Design review of the part built by this model. Coordinates are the model's own, in mm. A direction names the side the tool comes from. Coordinates: 2 decimals unless noted, no trailing zeros. Loops run counter-clockwise (first coordinate to the right, second up) from the corner with the lowest first, then second, coordinate; pieces in that order, holes last. Notation, with made-up numbers: M -35.75,-15.5 L -28.75,-15.5 A17 ccw -28.75,-11.5 Z; hole C 9,2.25 d4. An arc over 180 degrees is marked long. Answer as a JSON object with one key per item and string values. Group by question number.
1. Draft analysis for pull direction Y (two halves, no side actions). For faces 6 (the conical face through (-9.51, 40.769, -2.812)), 7 (the cylindrical face through (-1.97, -27.01, -24.85)), 8 (the flat face through (-20.3, 30, -2)), state which applies: +Y half, -Y half, draft (parallel to the pull), parting line (faces both ways), or undercut.
2. To check wall thickness, follow probe 1 along X at (y, z) = (-3.3, -10.15); probe 2 along X at (y, z) = (-3.5, -46); probe 3 along Z at (x, y) = (-19.5, 35). State the ranges of each line that lie inside material, in increasing order.
3. Consider section C-C (z = -17.5). State the section outline as (x, y) points, then the cut area to 3 significant figures.
4. Machinability: for faces 1 (the flat face through (-42, -24, -2)), 2 (the flat face through (-4, -31, -18)), 3 (the flat face through (-14, 25, -4)), 4 (the flat face through (-2, 30, -22)), 5 (the flat face through (-2, -24, -43)), which of the approach directions +Z, -Z, +X, -X, +Y, -Y give a long, thin tool a straight path to every point of the face, cutting with its end or side? Answer none if there is none.
5. Consider section B-B (x = -32). State the section outline as (y, z) points, then the cut area to 3 significant figures.
6. Insertion check: pin 1 (2 mm diameter, centred on x = -14.5, z = -8, fed in from -Y); pin 2 (1.2 mm diameter, centred on x = -10.15, z = -46, fed in from -Y); pin 3 (2.5 mm diameter, centred on x = -9.5, y = 42, fed in from +Z); pin 4 (12 mm diameter, centred on x = -16.5, y = -45, fed in from -Z). Each pin has a flat end and moves straight along its axis. Give the tip position at first contact, or say it passes through.
7. Consider section A-A (z = -38.5). State the section outline as (x, y) points, then the cut area to 3 significant figures.
from build123d import *

# Parameters (mm, degrees)
SKETCH1_W                    = 33.7
SKETCH1_H                    = 20.3
SKETCH1_W_2                  = 20.3
SKETCH1_H_2                  = 33.7
BOSS_EXTRUDE1_DEPTH          = 24
SHELL1_T                     = -4
SKETCH2_R                    = 1
CUT_EXTRUDE1_DEPTH           = 24
SKETCH3_R                    = 4.2
CUT_EXTRUDE2_DEPTH           = 3
CUT_EXTRUDE2_DRAFT           = -45
CUT_EXTRUDE2_PROFILE_2_DEPTH = 3
CUT_EXTRUDE2_PROFILE_2_DRAFT = -45
SKETCH4_W                    = 20.3
SKETCH4_H                    = 22
BOSS_EXTRUDE2_DEPTH          = 50
SHELL2_T                     = -4
CUT_EXTRUDE3_REACH           = 93.28
SKETCH5_R                    = 1
SKETCH6_R                    = 4.2
CUT_EXTRUDE4_DEPTH           = 3
CUT_EXTRUDE4_DRAFT           = -45
CUT_EXTRUDE5_REACH           = 93.28
SKETCH7_R                    = 1
SKETCH8_R                    = 4.2
CUT_EXTRUDE6_DEPTH           = 3
CUT_EXTRUDE6_DRAFT           = -45
FILLET1_R                    = 10
BOSS_EXTRUDE3_DEPTH          = 50
MIRROR4_COPY_1_SKETCH_R      = 4.2
MIRROR4_COPY_1_DEPTH         = 3
MIRROR4_COPY_1_DRAFT         = -45
MIRROR4_COPY_2_SKETCH_R      = 4.2
MIRROR4_COPY_2_DEPTH         = 3
MIRROR4_COPY_2_DRAFT         = -45
FILLET2_R                    = 10


with BuildPart() as part:
    # Sketch1 → Boss-Extrude1 (new body)
    with BuildSketch(Plane(origin=(0, 0, 0), x_dir=(1, 0, 0), z_dir=(0, 1, 0))):
        with Locations((-37.15, 10.15)):
            Rectangle(SKETCH1_W, SKETCH1_H)
        with Locations((-10.15, 10.15)):
            Rectangle(SKETCH1_W_2, SKETCH1_H)
        with Locations((-10.15, 37.15)):
            Rectangle(SKETCH1_W_2, SKETCH1_H_2)
    extrude(amount=-BOSS_EXTRUDE1_DEPTH)

    # Shell1
    shell1_openings = [part.faces().sort_by_distance(p)[0] for p in [
        (-53.236324676, -24, -10.15),
        (-54, -12, -10.15),
        (-37.15, -12, -20.3),
        (-20.3, -12, -37.15),
        (-10.15, -12, -54),
    ]]
    offset(amount=SHELL1_T, openings=shell1_openings, kind=Kind.INTERSECTION)

    # Sketch2 → Cut-Extrude1 (cut)
    with BuildSketch(Plane(origin=(0, 0, 0), x_dir=(1, 0, 0), z_dir=(0, 1, 0))):
        with Locations(Location((-10.15, 46, 0), (0, 0, 270))):
            Circle(SKETCH2_R)
        with Locations(Location((-46, 10.15, 0), (0, 0, 270))):
            Circle(SKETCH2_R)
    extrude(amount=-CUT_EXTRUDE1_DEPTH, mode=Mode.SUBTRACT)


with BuildPart() as cut_extrude2_tool:
    # Sketch3 → Cut-Extrude2 (with draft: the straight prism first)
    with BuildSketch(Plane(origin=(0, 0, 0), x_dir=(1, 0, 0), z_dir=(0, 1, 0))):
        with Locations((-46, 10.15)):
            Circle(SKETCH3_R)
    extrude(amount=-CUT_EXTRUDE2_DEPTH)
    # Cut-Extrude2: the draft: its side faces are tilted about the plane it starts from
    cut_extrude2_sides = [cut_extrude2_tool.faces().sort_by_distance(p)[0] for p in [
        (-50.2, -1.5, -10.15),
    ]]
    draft(cut_extrude2_sides, Plane(origin=(0, 0, 0), x_dir=(1, 0, 0), z_dir=(0, 1, 0)), CUT_EXTRUDE2_DRAFT)


with BuildPart() as part_1:
    add(part.part)

    # Cut-Extrude2: cut by cut_extrude2_tool
    add(cut_extrude2_tool.part, mode=Mode.SUBTRACT)


with BuildPart() as cut_extrude2_profile_2_tool:
    # Sketch3 → Cut-Extrude2 profile 2 (with draft: the straight prism first)
    with BuildSketch(Plane(origin=(0, 0, 0), x_dir=(1, 0, 0), z_dir=(0, 1, 0))):
        with Locations((-10.15, 46)):
            Circle(SKETCH3_R)
    extrude(amount=-CUT_EXTRUDE2_PROFILE_2_DEPTH)
    # Cut-Extrude2 profile 2: the draft: its side faces are tilted about the plane it starts from
    cut_extrude2_profile_2_sides = [cut_extrude2_profile_2_tool.faces().sort_by_distance(p)[0] for p in [
        (-14.35, -1.5, -46),
    ]]
    draft(cut_extrude2_profile_2_sides, Plane(origin=(0, 0, 0), x_dir=(1, 0, 0), z_dir=(0, 1, 0)), CUT_EXTRUDE2_PROFILE_2_DRAFT)


with BuildPart() as part_2:
    add(part_1.part)

    # Cut-Extrude2 profile 2: cut by cut_extrude2_profile_2_tool
    add(cut_extrude2_profile_2_tool.part, mode=Mode.SUBTRACT)


with BuildPart() as body_2:
    # Sketch4 → Boss-Extrude2 (new body)
    with BuildSketch(Plane(origin=(0, 0, 0), x_dir=(1, 0, 0), z_dir=(0, 1, 0))):
        with Locations((-10.15, 11)):
            Rectangle(SKETCH4_W, SKETCH4_H)
    extrude(amount=BOSS_EXTRUDE2_DEPTH)

    # Shell2
    shell2_openings = [body_2.faces().sort_by_distance(p)[0] for p in [
        (-10.15, 50, -11),
        (-10.15, 0, -11),
        (-20.3, 25, -11),
        (-10.15, 25, -22),
    ]]
    offset(amount=SHELL2_T, openings=shell2_openings, kind=Kind.INTERSECTION)


with BuildPart() as part_3:
    add(part_2.part)

    # Combine1: union body 2
    add(body_2.part)

    # Sketch5 → Cut-Extrude3 (cut, up to next)
    with BuildSketch(Plane.XY, mode=Mode.PRIVATE) as cut_extrude3_sk1:
        with Locations((-10.15, 42)):
            Circle(SKETCH5_R)
    cut_extrude3_tool1 = extrude(cut_extrude3_sk1.sketch, amount=-CUT_EXTRUDE3_REACH, mode=Mode.PRIVATE) & part_3.part
    cut_extrude3 = cut_extrude3_tool1.solids().sort_by_distance((-10.15, 42, 0))[0]
    add(cut_extrude3, mode=Mode.SUBTRACT)


with BuildPart() as cut_extrude4_tool:
    # Sketch6 → Cut-Extrude4 (with draft: the straight prism first)
    with BuildSketch(Plane.XY):
        with Locations((-10.15, 42)):
            Circle(SKETCH6_R)
    extrude(amount=-CUT_EXTRUDE4_DEPTH)
    # Cut-Extrude4: the draft: its side faces are tilted about the plane it starts from
    cut_extrude4_sides = [cut_extrude4_tool.faces().sort_by_distance(p)[0] for p in [
        (-14.35, 42, -1.5),
    ]]
    draft(cut_extrude4_sides, Plane.XY, CUT_EXTRUDE4_DRAFT)


with BuildPart() as part_4:
    add(part_3.part)

    # Cut-Extrude4: cut by cut_extrude4_tool
    add(cut_extrude4_tool.part, mode=Mode.SUBTRACT)

    # Sketch7 → Cut-Extrude5 (cut, up to next)
    with BuildSketch(Plane(origin=(0, 0, 0), x_dir=(0, 0, -1), z_dir=(1, 0, 0)), mode=Mode.PRIVATE) as cut_extrude5_sk1:
        with Locations((11, 20)):
            Circle(SKETCH7_R)
    cut_extrude5_tool1 = extrude(cut_extrude5_sk1.sketch, amount=-CUT_EXTRUDE5_REACH, mode=Mode.PRIVATE) & part_4.part
    cut_extrude5 = cut_extrude5_tool1.solids().sort_by_distance((0, 20, -11))[0]
    add(cut_extrude5, mode=Mode.SUBTRACT)


with BuildPart() as cut_extrude6_tool:
    # Sketch8 → Cut-Extrude6 (with draft: the straight prism first)
    with BuildSketch(Plane(origin=(0, 0, 0), x_dir=(0, 0, -1), z_dir=(1, 0, 0))):
        with Locations((11, 20)):
            Circle(SKETCH8_R)
    extrude(amount=-CUT_EXTRUDE6_DEPTH)
    # Cut-Extrude6: the draft: its side faces are tilted about the plane it starts from
    cut_extrude6_sides = [cut_extrude6_tool.faces().sort_by_distance(p)[0] for p in [
        (-1.5, 20, -6.8),
    ]]
    draft(cut_extrude6_sides, Plane(origin=(0, 0, 0), x_dir=(0, 0, -1), z_dir=(1, 0, 0)), CUT_EXTRUDE6_DRAFT)


with BuildPart() as part_5:
    add(part_4.part)

    # Cut-Extrude6: cut by cut_extrude6_tool
    add(cut_extrude6_tool.part, mode=Mode.SUBTRACT)

    # Fillet1
    fillet1_edges = [part_5.edges().sort_by_distance(p)[0] for p in [
        (-2, 0, -22),
        (-20.3, 0, -2),
    ]]
    fillet(fillet1_edges, radius=FILLET1_R)

    # Sketch9 → Boss-Extrude3 (add)
    with BuildSketch(Plane.XZ.offset(24)):
        Polygon((-4, -4), (-4, -22), (0, -22), (0, 0), (-20.3, 0), (-20.3, -4), align=None)
    extrude(amount=BOSS_EXTRUDE3_DEPTH)

    # Mirror4: Cut-Extrude3, Cut-Extrude5 across plane
    add(cut_extrude3.mirror(Plane(origin=(0, -12, 0), x_dir=(0, 0, 1), z_dir=(0, -1, 0))), mode=Mode.SUBTRACT)
    add(cut_extrude5.mirror(Plane(origin=(0, -12, 0), x_dir=(0, 0, 1), z_dir=(0, -1, 0))), mode=Mode.SUBTRACT)


with BuildPart() as mirror4_copy_1_tool:
    # Mirror4 copy 1 sketch → Mirror4 copy 1 (with draft: the straight prism first)
    with BuildSketch(Plane(origin=(0, -24, 0), x_dir=(1, 0, 0), z_dir=(0, 0, 1))):
        with Locations((-10.15, -42)):
            Circle(MIRROR4_COPY_1_SKETCH_R)
    extrude(amount=-MIRROR4_COPY_1_DEPTH)
    # Mirror4 copy 1: the draft: its side faces are tilted about the plane it starts from
    mirror4_copy_1_sides = [mirror4_copy_1_tool.faces().sort_by_distance(p)[0] for p in [
        (-14.35, -66, -1.5),
    ]]
    draft(mirror4_copy_1_sides, Plane(origin=(0, -24, 0), x_dir=(1, 0, 0), z_dir=(0, 0, 1)), MIRROR4_COPY_1_DRAFT)


with BuildPart() as part_6:
    add(part_5.part)

    # Mirror4 copy 1: cut by mirror4_copy_1_tool
    add(mirror4_copy_1_tool.part, mode=Mode.SUBTRACT)


with BuildPart() as mirror4_copy_2_tool:
    # Mirror4 copy 2 sketch → Mirror4 copy 2 (with draft: the straight prism first)
    with BuildSketch(Plane(origin=(0, -24, 0), x_dir=(0, 0, -1), z_dir=(1, 0, 0))):
        with Locations((11, -20)):
            Circle(MIRROR4_COPY_2_SKETCH_R)
    extrude(amount=-MIRROR4_COPY_2_DEPTH)
    # Mirror4 copy 2: the draft: its side faces are tilted about the plane it starts from
    mirror4_copy_2_sides = [mirror4_copy_2_tool.faces().sort_by_distance(p)[0] for p in [
        (-1.5, -44, -6.8),
    ]]
    draft(mirror4_copy_2_sides, Plane(origin=(0, -24, 0), x_dir=(0, 0, -1), z_dir=(1, 0, 0)), MIRROR4_COPY_2_DRAFT)


with BuildPart() as part_7:
    add(part_6.part)

    # Mirror4 copy 2: cut by mirror4_copy_2_tool
    add(mirror4_copy_2_tool.part, mode=Mode.SUBTRACT)

    # Fillet2
    fillet2_edges = [part_7.edges().sort_by_distance(p)[0] for p in [
        (-2, -24, -22),
        (-20.3, -24, -2),
    ]]
    fillet(fillet2_edges, radius=FILLET2_R)


solid = part_7.part
Findings below:
{
 "1": {"face 6": "undercut", "face 7": "-Y half", "face 8": "draft"},
 "2": {"probe 1": "x = -54 to -47, -45 to 0", "probe 2": "x = -20.3 to -11.15, -9.15 to 0", "probe 3": "z = -4 to 0"},
 "3": {"outline": "M -54,-4 L -4,-4 L -4,-74 L 0,-74 L 0,50 L -4,50 L -4,0 L -54,0 Z", "area": "696 mm^2"},
 "4": {"face 1": "+Z, -Z, -X, -Y", "face 2": "-Z, -X, -Y", "face 3": "-Z, -X, +Y", "face 4": "-Z, +X, -X, +Y", "face 5": "-Z, +X, -X, -Y"},
 "5": {"outline": "M -24,-4 L -4,-4 L -4,-20.3 L 0,-20.3 L 0,0 L -24,0 Z", "area": "161 mm^2"},
 "6": {"pin 1": "stops at y = -4", "pin 2": "passes through", "pin 3": "stops at z = -2.3", "pin 4": "stops at z = -4"},
 "7": {"outline": "M -20.3,-4 L -4,-4 L -4,-24 L 0,-24 L 0,0 L -20.3,0 Z", "area": "161 mm^2"}
}
